Read the model definition and answer for the solid it produces. Units are mm, in the model's axes. A direction names the side the tool comes from. Coordinates: 2 decimals unless noted, no trailing zeros. Write each loop counter-clockwise with the first axis right and the second up, starting at its lowest first coordinate (ties: lowest second). Pieces come first, ordered by that corner, then holes. Notation, with made-up numbers: (21.5, 54.5) -> (52.5, 54.5) arc R21 ccw to (52.5, 88.5) -> close; hole circle Ø8 at (-25.5, 7.25). An arc over 180 degrees is marked (long way). Use CSV: the item, a comma, the result in double quotes.
from build123d import *

# Parameters (mm, degrees)
BOSS_EXTRUDE1_DEPTH      = 11
BOSS_EXTRUDE2_DEPTH      = 16.4
BOSS_EXTRUDE2_DEPTH_BACK = 17.5
SKETCH2_R                = 3.25
SKETCH3_R                = 2.3
CUT_EXTRUDE1_DEPTH       = 28.9
SKETCH4_R                = 3.25
BOSS_EXTRUDE3_DEPTH      = 16.5
SKETCH5_R                = 2.3
CUT_EXTRUDE2_DEPTH       = 28
BOSS_EXTRUDE4_START      = -20.5
BOSS_EXTRUDE4_DEPTH      = 21
SKETCH8_R                = 9.5
BOSS_EXTRUDE5_DEPTH      = 32
SKETCH10_R               = 2.25
BOSS_EXTRUDE6_DEPTH      = 2.5
FILLET1_R                = 2


with BuildPart() as part:
    # Sketch1 → Boss-Extrude1 (new body)
    with BuildSketch(Plane(origin=(0, 0, 0), x_dir=(1, 0, 0), z_dir=(0, 1, 0))):
        with BuildLine():
            Line((2.5, 0), (17.5, 0))
            ThreePointArc((17.5, 0), (19.267766953, 0.732233047), (20, 2.5))
            Line((20, 2.5), (20, 17.5))
            ThreePointArc((20, 17.5), (19.267766953, 19.267766953), (17.5, 20))
            Line((17.5, 20), (2.5, 20))
            ThreePointArc((2.5, 20), (0.732233047, 19.267766953), (0, 17.5))
            Line((0, 17.5), (0, 2.5))
            ThreePointArc((0, 2.5), (0.732233047, 0.732233047), (2.5, 0))
        make_face()
    extrude(amount=BOSS_EXTRUDE1_DEPTH)

    # Sketch2 → Boss-Extrude2 (add, two sides: drawn at the far end of the back side and taken through both)
    with BuildSketch(Plane.XY.offset(-BOSS_EXTRUDE2_DEPTH_BACK)):
        with Locations((10, 0)):
            Circle(SKETCH2_R)
    extrude(amount=BOSS_EXTRUDE2_DEPTH + BOSS_EXTRUDE2_DEPTH_BACK)

    # Sketch3 → Cut-Extrude1 (cut)
    with BuildSketch(Plane.XY.offset(16.4)):
        with Locations((10, 0)):
            Circle(SKETCH3_R)
    extrude(amount=-CUT_EXTRUDE1_DEPTH, mode=Mode.SUBTRACT)

    # Sketch4 → Boss-Extrude3 (add)
    with BuildSketch(Plane(origin=(0, 0, -20), x_dir=(-1, 0, 0), z_dir=(0, 0, -1))):
        with Locations(Location((-10, 4.25, 0), (0, 0, 180))):
            Circle(SKETCH4_R)
    extrude(amount=BOSS_EXTRUDE3_DEPTH)

    # Sketch5 → Cut-Extrude2 (cut)
    with BuildSketch(Plane(origin=(0, 0, -36.5), x_dir=(-1, 0, 0), z_dir=(0, 0, -1))):
        with Locations((-10, 4.25)):
            Circle(SKETCH5_R)
    extrude(amount=-CUT_EXTRUDE2_DEPTH, mode=Mode.SUBTRACT)

    # Sketch7 → Boss-Extrude4 (add)
    with BuildSketch(Plane(origin=(20, 0, 0), x_dir=(0, 0, -1), z_dir=(1, 0, 0)).offset(BOSS_EXTRUDE4_START)):
        with BuildLine():
            Line((-1, 11), (21, 11))
            Line((21, 11), (21, 10))
            Line((21, 10), (23, 10))
            Line((23, 10), (23, 45))
            ThreePointArc((23, 45), (22.414213562, 46.414213562), (21, 47))
            Line((21, 47), (-1, 47))
            ThreePointArc((-1, 47), (-2.414213562, 46.414213562), (-3, 45))
            Line((-3, 45), (-3, 10))
            Line((-3, 10), (-1, 10))
            Line((-1, 10), (-1, 11))
        make_face()
        with BuildLine():
            Line((-0.5, 13), (20.5, 13))
            ThreePointArc((20.5, 13), (20.853553391, 13.146446609), (21, 13.5))
            Line((21, 13.5), (21, 44.5))
            ThreePointArc((21, 44.5), (20.853553391, 44.853553391), (20.5, 45))
            Line((20.5, 45), (-0.5, 45))
            ThreePointArc((-0.5, 45), (-0.853553391, 44.853553391), (-1, 44.5))
            Line((-1, 44.5), (-1, 13.5))
            ThreePointArc((-1, 13.5), (-0.853553391, 13.146446609), (-0.5, 13))
        make_face(mode=Mode.SUBTRACT)
    extrude(amount=BOSS_EXTRUDE4_DEPTH)

    # Sketch8 → Boss-Extrude5 (add)
    with BuildSketch(Plane(origin=(0, 13, 0), x_dir=(1, 0, 0), z_dir=(0, 1, 0))):
        with Locations(Location((10, 10, 0), (0, 0, 90))):
            Circle(SKETCH8_R)
    extrude(amount=BOSS_EXTRUDE5_DEPTH)

    # Sketch10 → Boss-Extrude6 (add)
    with BuildSketch(Plane(origin=(20.5, 0, 0), x_dir=(0, 0, -1), z_dir=(1, 0, 0))):
        Polygon((-13, 19), (33, 19), (33, 13), (21, 13), (21, 11), (-1, 11), (-1, 13), (-13, 13), align=None)
        with Locations((-9, 16)):
            Circle(SKETCH10_R, mode=Mode.SUBTRACT)
        with Locations((28.999999979, 15.998723468)):
            Circle(SKETCH10_R, mode=Mode.SUBTRACT)
    extrude(amount=BOSS_EXTRUDE6_DEPTH)

    # Fillet1
    fillet1_edges = [part.edges().sort_by_distance(p)[0] for p in [
        (23, 11, -10),
    ]]
    fillet(fillet1_edges, radius=FILLET1_R)


solid = part.part
1. A cutting plane is placed at D-D (z = -10). Give the vertices of the cut face in (x, y) (3 decimals).
Solutions:
outline,"(-0.5, 11) -> (0, 11) -> (0, 0) -> (6.75, 0) arc R3.25 ccw to (13.25, 0) -> (20, 0) -> (20, 11) -> (21, 11) arc R2 ccw to (23, 13) -> (23, 19) -> (20.5, 19) -> (20.5, 13) -> (19.5, 13) -> (19.5, 45) -> (20.5, 45) -> (20.5, 47) -> (-0.5, 47) -> (-0.5, 45) -> (0.5, 45) -> (0.5, 13) -> (-0.5, 13) -> close; hole (9.12, 2.125) arc R2.3 ccw (long way) to (10.88, 2.125) arc R2.3 ccw (long way) to start"
2. A cutting plane is placed at C-C (x = 10). Give the number of separate pieces and of enclosed holes in the cut face, and give its area (3 significant figures).
Solutions:
separate pieces,"2"
enclosed holes,"2"
area,"1,070 mm^2"
3. A cutting plane is placed at A-A (z = 9). Give the vertices of the cut face in (x, y).
Solutions:
outline,"circle Ø6.5 at (10, 0); (20.5, 13) -> (23, 13) -> (23, 13.75) -> (20.5, 13.75) -> close; (20.5, 18.25) -> (23, 18.25) -> (23, 19) -> (20.5, 19) -> close; hole circle Ø4.6 at (10, 0)"
4. Each of these flat-tipped pins is pushed along its axis until it touches: pin 1 Ø3 at (y, z) = (36, 4) entering from -X; pin 2 Ø12 at (x, y) = (8, 32) entering from +Z; pin 3 Ø3.5 at (x, y) = (12, 7.5) entering from +Z; pin 4 Ø2.5 at (x, y) = (10, -1) entering from -Z. Where does it stop, or does it pass through?
Solutions:
pin 1,"stops at x = -0.5"
pin 2,"stops at z = 3"
pin 3,"stops at z = 0"
pin 4,"stops at z = -20"
5. A tool of negligible diameter and unlimited length cuts with its end or side. For faces 1 (the flat face through (20.5, 12, -22)), 2 (the flat face through (20.5, 17.4, 6.8)), 3 (the flat face through (20.5, 16, -10)), 4 (the flat face through (22, 13, 7)), 5 (the cylindrical face through (9.295, -3.173, 2.979)), from which of +Z, -Z, +X, -X, +Y, -Y can it reach the whole face along a straight path? Write none if from no direction.
Solutions:
face 1,"-Z, +X, -Y"
face 2,"+Z, -X, +Y, -Y"
face 3,"none"
face 4,"+Z, +X, -Y"
face 5,"+Z"
6. For a pull along Z with two mould halves and no side action, classify faces 6 (the flat face through (7.5, 45, -19.5)), 7 (the cylindrical face through (9.85, 46.43, 2.4)), 8 (the cylindrical face through (21.732, 13.804, 9.488)), 9 (the flat face through (10, 10, -22)) as pulls with the +Z half, pulls with the -Z half, needs draft (parallel to the pull), parting line crosses it, or undercut.
Solutions:
face 6,"undercut"
face 7,"pulls with the +Z half"
face 8,"undercut"
face 9,"needs draft"
7. A cutting plane is placed at B-B (y = 40). Give the vertices of the cut face in (x, z), and give its area (3 significant figures).
Solutions:
outline,"(-0.5, -23) -> (20.5, -23) -> (20.5, -21) -> (-0.5, -21) -> close; (-0.5, 1) -> (20.5, 1) -> (20.5, 3) -> (-0.5, 3) -> close; circle Ø19 at (10, -10)"
area,"368 mm^2"
8. Find the intervals of material crossed by line 1 along Y through (x, z) = (10, -4.25); line 2 along X through (y, z) = (0, 10.25); line 3 along Y through (x, z) = (10, -29.75), in increasing order.
Solutions:
line 1,"y = -3.25 to -2.3, 2.3 to 47"
line 2,"x = 6.75 to 7.7, 12.3 to 13.25"
line 3,"y = 1 to 1.95, 6.55 to 7.5"
